Can you work these out from the model? Positions are in its coordinate system, mm. Face numbers are marked on the shaded views. Give positions to 0.01 mm unless a question says otherwise; leave off trailing zeros. Order: outer loops, then holes, each group sorted by start corner. A loop starts at its lowest first (then second) coordinate and runs counter-clockwise, first axis right, second up. Notation, with made-up numbers: M 38,53.25 L 82,53.25 A29 ccw 82,74.25 Z; hole C 33,-15.75 d1. An arc over 180 degrees is marked long. Write each question's results on one line, items separated by ' | '.
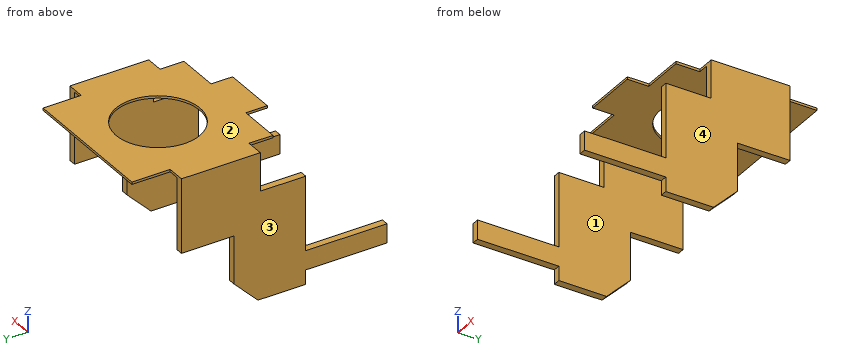
from build123d import *

# Parameters (mm, degrees)
SKETCH1_R                = 1.75
BOSS_EXTRUDE1_DEPTH      = 0.1
SKETCH2_W                = 0.3
SKETCH2_H                = 3.3
BOSS_EXTRUDE2_DEPTH      = 3
BOSS_EXTRUDE3_DEPTH      = 3
BOSS_EXTRUDE3_DEPTH_BACK = 1.5
SKETCH3_W                = 0.3
SKETCH3_H                = 3
CUT_EXTRUDE1_DEPTH       = 11.725320508
CUT_EXTRUDE1_DEPTH_BACK  = 11.725320508
SKETCH6_W                = 0.3
SKETCH6_H                = 0.8
BOSS_EXTRUDE4_DEPTH      = 3.4


with BuildPart() as part:
    # Sketch1 → Boss-Extrude1 (new body)
    with BuildSketch(Plane.XY):
        Polygon((1.8, 0), (1.8, -0.9), (4.1, -0.9), (4.1, 0), (5.9, 0), (5.9, 1), (6.65, 1), (6.65, 4.3), (5.9, 4.3), (5.9, 5.9), (0, 5.9), (0, 4.3), (-0.75, 4.3), (-0.75, 1), (0, 1), (0, 0), align=None)
        with Locations((2.95, 2.95)):
            Circle(SKETCH1_R, mode=Mode.SUBTRACT)
    extrude(amount=BOSS_EXTRUDE1_DEPTH)

    # Sketch2 → Boss-Extrude2 (add)
    with BuildSketch(Plane(origin=(0, 0, 0), x_dir=(-1, 0, 0), z_dir=(0, 0, -1))):
        with Locations((-6.5, 2.65)):
            Rectangle(SKETCH2_W, SKETCH2_H)
        with Locations((0.6, 2.65)):
            Rectangle(SKETCH2_W, SKETCH2_H)
    extrude(amount=BOSS_EXTRUDE2_DEPTH)

    # Sketch3 → Boss-Extrude3 (add, two sides: drawn at the far end of the back side and taken through both)
    with BuildSketch(Plane(origin=(0, 0, -3), x_dir=(-1, 0, 0), z_dir=(0, 0, -1)).offset(-BOSS_EXTRUDE3_DEPTH_BACK)):
        with Locations((0.6, 0.6)):
            Rectangle(SKETCH3_W, SKETCH3_H)
        with Locations((-6.5, 0.6)):
            Rectangle(SKETCH3_W, SKETCH3_H)
    extrude(amount=BOSS_EXTRUDE3_DEPTH + BOSS_EXTRUDE3_DEPTH_BACK)

    # Sketch5 → Cut-Extrude1 (cut, two sides: drawn at the far end of the back side and taken through both)
    with BuildSketch(Plane(origin=(0, 0, 0), x_dir=(0, 0, -1), z_dir=(1, 0, 0)).offset(-CUT_EXTRUDE1_DEPTH_BACK)):
        Polygon((5, 2.1), (6, 1.1), (6, 2.1), align=None)
    extrude(amount=CUT_EXTRUDE1_DEPTH + CUT_EXTRUDE1_DEPTH_BACK, mode=Mode.SUBTRACT)

    # Sketch6 → Boss-Extrude4 (add)
    with BuildSketch(Plane.XZ.offset(0.9)):
        with Locations((-0.6, -5)):
            Rectangle(SKETCH6_W, SKETCH6_H)
        with Locations((6.5, -5)):
            Rectangle(SKETCH6_W, SKETCH6_H)
    extrude(amount=BOSS_EXTRUDE4_DEPTH)


solid = part.part
(1) Will these pins go through, and if not, where does the flat tip stop? P1, Ø0.8, axis at x = -0.5, z = -0.5, coming from the -Y side; P2, Ø0.8, axis at x = -0.5, z = -1, coming from the +Y side.
Data:
P1: stops at y = 1 | P2: stops at y = 4.3
(2) Imagine slicing it at B-B, the plane y = -1.5. Write out the boundary of the cut face in (x, z).
Data:
outline: M -0.75,-5.4 L -0.45,-5.4 L -0.45,-4.6 L -0.75,-4.6 Z; M 6.35,-5.4 L 6.65,-5.4 L 6.65,-4.6 L 6.35,-4.6 Z
(3) We'd pull the mould along X, two halves only. Please class the marked faces 1, 2, 3 and 4: +X half, -X half, draft (parallel to the pull), parting line (faces both ways), or undercut.
Data:
face 1: undercut | face 2: draft | face 3: -X half | face 4: +X half
(4) Imagine slicing it at A-A, the plane z = -1.25. Write out the boundary of the cut face in (x, y).
Data:
outline: M -0.75,1 L -0.45,1 L -0.45,4.3 L -0.75,4.3 Z; M 6.35,1 L 6.65,1 L 6.65,4.3 L 6.35,4.3 Z
(5) I need wall thicknesses on L1, parallel to X at y = 3.75, z = -1.25. Which ranges of the line are inside material? Lowest first, please. Write a range as from..to.
Data:
L1: x = -0.75..-0.45, 6.35..6.65
(6) Imagine slicing it at D-D, the plane y = 2.95. Write out the boundary of the cut face in (x, z).
Data:
outline: M -0.75,-3 L -0.45,-3 L -0.45,0 L 1.2,0 L 1.2,0.1 L -0.75,0.1 Z; M 4.7,0 L 6.35,0 L 6.35,-3 L 6.65,-3 L 6.65,0.1 L 4.7,0.1 Z
(7) Imagine slicing it at C-C, the plane y = 0.5. Write out the boundary of the cut face in (x, z).
Data:
outline: M -0.75,-6 L -0.45,-6 L -0.45,-1.5 L -0.75,-1.5 Z; M 0,0 L 5.9,0 L 5.9,0.1 L 0,0.1 Z; M 6.35,-6 L 6.65,-6 L 6.65,-1.5 L 6.35,-1.5 Z
